Autodesk Inventor part; units mm, degrees
ref_plane "YZ Plane" through (0, 0, 0) normal (1, 0, 0) x (0, 1, 0)
ref_plane "XZ Plane" through (0, 0, 0) normal (0, 1, 0) x (-1, 0, 0)
ref_plane "XY Plane" through (0, 0, 0) normal (0, 0, 1) x (1, 0, 0)
sketch "Sketch1" plane through (0, 0, 0) normal (0, 0, 1) x (1, 0, 0)
  line L0 (-42.7621, 33.3504) -> (37.2379, 33.3504)
  line L1 (37.2379, 33.3504) -> (37.2379, -26.6496)
  line L2 (37.2379, -26.6496) -> (-42.7621, -26.6496)
  line L3 (-42.7621, -26.6496) -> (-42.7621, 33.3504)
  point P0 (0, 0)
  dimension "d0" = 80
  dimension "d1" = 60
extrude "Extrusion1" add sketch "Sketch1" along normal blind 50
sketch "Sketch2" plane through (0, 0, 50) normal (0, 0, 1) x (1, 0, 0)
  line L0 (-30.0743, 35.3951) -> (-16.0743, 35.3951)
  line L1 (-16.0743, 35.3951) -> (-16.0743, 26.3951)
  line L2 (-16.0743, 26.3951) -> (-10.5743, 26.3951)
  line L3 (-10.5743, 26.3951) -> (-10.5743, 16.3951)
  line L4 (-10.5743, 16.3951) -> (-35.5743, 16.3951)
  line L5 (-35.5743, 16.3951) -> (-35.5743, 26.3951)
  line L6 (-35.5743, 26.3951) -> (-30.0743, 26.3951)
  line L7 (-30.0743, 26.3951) -> (-30.0743, 35.3951)
  point P0 (0, 0)
  point P1 (-23.0743, 35.3951)
  dimension "d4" = 14
  dimension "d5" = 25
  dimension "d6" = 10
  dimension "d7" = 9
  dimension "d8" = 7
  dimension "d9" = 12.5
extrude "Extrusion2" cut sketch "Sketch2" against normal blind 50
sketch "Sketch3" plane through (0, 0, 50) normal (0, 0, 1) x (1, 0, 0)
  line L0 (25.1509, 34.1359) -> (32.1509, 34.1359)
  line L1 (32.1509, 34.1359) -> (32.1509, 29.8137)
  line L2 (32.1509, 29.8137) -> (33.5651, 28.3995)
  line L3 (33.5651, 28.3995) -> (32.1509, 26.9853)
  line L4 (32.1509, 26.9853) -> (30.0002, 29.1359)
  line L5 (30.0002, 29.1359) -> (25.1509, 29.1359)
  line L6 (25.1509, 34.1359) -> (25.1509, 29.1359) construction
  line L7 (25.1509, 34.1359) -> (18.1509, 34.1359)
  line L8 (18.1509, 34.1359) -> (18.1509, 29.8137)
  line L9 (18.1509, 29.8137) -> (16.7366, 28.3995)
  line L10 (16.7366, 28.3995) -> (18.1509, 26.9853)
  line L11 (18.1509, 26.9853) -> (20.3015, 29.1359)
  line L12 (20.3015, 29.1359) -> (25.1509, 29.1359)
  point P0 (0, 0)
  dimension "d12" = 7
  dimension "d13" = 5
  dimension "d14" = 2
  dimension "d15" = 2
  dimension "d16" = 135
  dimension "d17" = 4.3222
extrude "Extrusion3" cut sketch "Sketch3" against normal blind 50
properties part number "PiesaSuportCanale"
Read the model definition and answer for the solid it produces. Units are mm, in the model's axes. A direction names the side the tool comes from. Coordinates: 2 decimals unless noted, no trailing zeros. Order: outer loops, then holes, each group sorted by start corner. A loop starts at its lowest first (then second) coordinate and runs counter-clockwise, first axis right, second up. Notation, with made-up numbers: (17, 52.25) -> (63, 52.25) arc R31 cw to (63, 91.25) -> close; hole circle Ø10 at (-38, -6.5). An arc over 180 degrees is marked (long way). Answer as a JSON object with one key per item and string values.
1) A tool of negligible diameter and unlimited length cuts with its end or side. For faces 4 (the face through (25, 29.136, 25)), 5 (the face through (37.238, 4, 25)), 6 (the face through (-23, 16.395, 25)), from which of +Z, -Z, +X, -X, +Y, -Y can it reach the whole face along a straight path? Write none if from no direction.
Model answer:
{"face 4": "+Z, -Z, +Y", "face 5": "+Z, -Z, +X, +Y, -Y", "face 6": "+Z, -Z"}
2) Consider line 1 along X through (y, z) = (16.5, 4.5); line 2 along X through (y, z) = (30.5, 28.5); line 3 along Y through (x, z) = (-25.5, 34). Determine where each line is inside the solid, lowest interval first. Write a range as from..to.
Model answer:
{"line 1": "x = -42.76..-35.57, -10.57..37.24", "line 2": "x = -42.76..-30.07, -16.07..18.15, 32.15..37.24", "line 3": "y = -26.65..16.4"}
3) A cutting plane is placed at C-C, the plane z = 30. Determine the outline of the cut face in (x, y), plus the area to 4 significant figures.
Model answer:
{"outline": "(-42.76, -26.65) -> (37.24, -26.65) -> (37.24, 33.35) -> (32.15, 33.35) -> (32.15, 29.81) -> (33.57, 28.4) -> (32.15, 26.99) -> (30, 29.14) -> (20.3, 29.14) -> (18.15, 26.99) -> (16.74, 28.4) -> (18.15, 29.81) -> (18.15, 33.35) -> (-16.07, 33.35) -> (-16.07, 26.4) -> (-10.57, 26.4) -> (-10.57, 16.4) -> (-35.57, 16.4) -> (-35.57, 26.4) -> (-30.07, 26.4) -> (-30.07, 33.35) -> (-42.76, 33.35) -> close", "area": "4,385 mm²"}
4) A cutting plane is placed at B-B, the plane y = 23.5. Determine the outline of the cut face in (x, z).
Model answer:
{"outline": "(-42.76, 0) -> (-35.57, 0) -> (-35.57, 50) -> (-42.76, 50) -> close; (-10.57, 0) -> (37.24, 0) -> (37.24, 50) -> (-10.57, 50) -> close"}
5) A cutting plane is placed at A-A, the plane x = -33.5. Determine the outline of the cut face in (y, z).
Model answer:
{"outline": "(-26.65, 0) -> (16.4, 0) -> (16.4, 50) -> (-26.65, 50) -> close; (26.4, 0) -> (33.35, 0) -> (33.35, 50) -> (26.4, 50) -> close"}
6) Each of these flat-tipped pins is pushed along its axis until it touches: pin 1 (6 mm diameter, centred on x = -21, y = 26, fed in from -Z); pin 2 (10.5 mm diameter, centred on x = 26, z = 28, fed in from +Y). Where does it stop, or does it pass through?
Model answer:
{"pin 1": "passes through", "pin 2": "stops at y = 29.14"}
7) The mould has two halves that part along Y. Classify faces 1 (the face through (18.151, 32, 25)), 2 (the face through (-35.574, 21, 25)), 3 (the face through (-37, 33.35, 25)): released by +Y, released by -Y, zero draft, split by the parting line, or undercut.
Model answer:
{"face 1": "zero draft", "face 2": "undercut", "face 3": "released by +Y"}
